Input: part model. Units: mm. Frame: model coordinates. Face numbers are marked on the shaded views. A direction names the side the tool comes from. Round coordinates to 2 decimals unless told otherwise and drop trailing zeros. Loops run counter-clockwise (first coordinate to the right, second up) from the corner with the lowest first, then second, coordinate; pieces in that order, holes last.
1) Section C-C, the plane x = 13. Return loops of the section in (y, z).
2) Section A-A, the plane y = 6.5. Return loops of the section in (x, z).
3) Access query for the marked faces 1, 2 and 3. Directions: +Z, -Z, +X, -X, +Y, -Y. A direction counts if a zero-diameter tool reaches every point of the face in a straight line with its end or side. Return the directions, or none.
4) Ray query, line 1 along Y through (x, z) = (28.5, 5.75); line 2 along X through (y, z) = (3, 23); line 3 along X through (y, z) = (13.25, 16.5). Return the intervals inside material, ascending.
5) Section B-B, the plane z = 18. Return loops of the section in (x, y), and give its area (3 significant figures).
6) First-contact query: pin 1 (2 mm diameter, centred on x = 17, z = 7.5, fed in from +Y); pin 2 (3 mm diameter, centred on y = -2, z = 12.5, fed in from -X); pin 3 (4 mm diameter, centred on x = 16.5, z = 23, fed in from -Y); pin 4 (1.5 mm diameter, centred on y = 13, z = 24, fed in from -X). Flat tips, straight axial feed; report the tip coordinate or a pass-through.
7) Section D-D, the plane y = 14.5. Return loops of the section in (x, z).
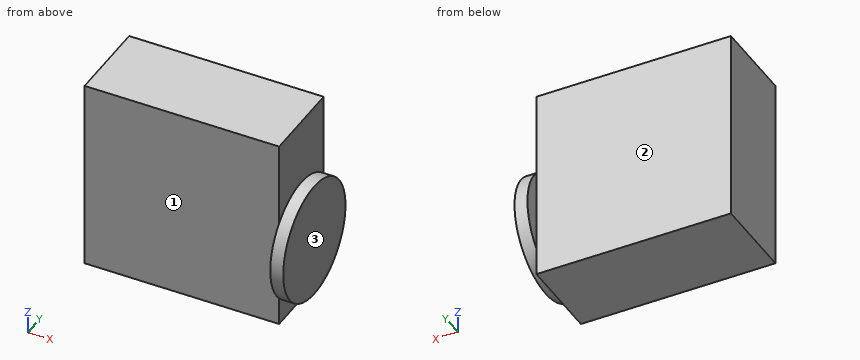
Autodesk Inventor part; units mm, degrees
ref_plane "YZ Plane" through (0, 0, 0) normal (1, 0, 0) x (0, 1, 0)
ref_plane "XZ Plane" through (0, 0, 0) normal (0, 1, 0) x (-1, 0, 0)
ref_plane "XY Plane" through (0, 0, 0) normal (0, 0, 1) x (1, 0, 0)
sketch "Esquisse1" plane through (0, 0, 0) normal (0, 1, 0) x (-1, 0, 0)
  line L0 (0, 0) -> (-30, 0)
  line L1 (-30, 0) -> (-30, 30)
  line L2 (-30, 30) -> (0, 30)
  line L3 (0, 30) -> (0, 0)
  dimension "d0" = 30
  dimension "d2" = 30
extrude "Extrusion1" add sketch "Esquisse1" along normal blind 13
sketch "Esquisse2" plane through (30, 0, 30) normal (1, 0, 0) x (0, 0, -1)
  circle A0 centre (19.3193, 6.5) radius 9.0917
extrude "Extrusion2" add sketch "Esquisse2" along normal blind 2
properties part number "moteur euger 16_03"
Final values:
1. outline: (0, 0) - (13, 0) - (13, 30) - (0, 30) - close
2. outline: (0, 0) - (30, 0) - (30, 1.59) - (32, 1.59) - (32, 19.77) - (30, 19.77) - (30, 30) - (0, 30) - close
3. face 1: +Z, -Z, -X, -Y
3. face 2: +Z, -Z, -X, +Y
3. face 3: +Z, -Z, +X, +Y, -Y
4. line 1: y = 0 to 13
4. line 2: x = 0 to 30
4. line 3: x = 30 to 32
5. outline: (0, 0) - (30, 0) - (30, 1.11) - (32, 1.11) - (32, 11.89) - (30, 11.89) - (30, 13) - (0, 13) - close
5. area: 412 mm2
6. pin 1: stops at y = 13
6. pin 2: stops at x = 30
6. pin 3: stops at y = 0
6. pin 4: stops at x = 0
7. outline: (30, 6.36) - (32, 6.36) - (32, 15) - (30, 15) - close
